Geometry check sheet. Reference: the model listing, model coordinates, mm. A direction names the side the tool comes from. Give positions to 0.01 mm unless a question says otherwise; leave off trailing zeros. Order: outer loops, then holes, each group sorted by start corner. A loop starts at its lowest first (then second) coordinate and runs counter-clockwise, first axis right, second up. Notation, with made-up numbers: M 26,-24.75 L 40,-24.75 A23 ccw 40,-15.75 Z; hole C 22,-21.5 d7. An arc over 180 degrees is marked long. One line per question, with ' | ' between items. Start each with the question number.
from build123d import *

# Parameters (mm, degrees)
SKETCH_1_W          = 50
SKETCH_1_H          = 50
EXTRUDE_1_DEPTH     = 3
SKETCH_2_W          = 50
SKETCH_2_H          = 50
SKETCH_2_W_2        = 44
SKETCH_2_H_2        = 44
EXTRUDE_2_DEPTH     = 17
SKETCH_3_W          = 4.5
SKETCH_3_H          = 2.5
CUT_EXTRUDE_1_DEPTH = 60.371710435
SKETCH_4_W          = 4.5
SKETCH_4_H          = 2.5
CUT_EXTRUDE_2_DEPTH = 60.371710435


with BuildPart() as part:
    # 草图1 → 凸台-拉伸1 (new body)
    with BuildSketch(Plane(origin=(0, 0, 0), x_dir=(1, 0, 0), z_dir=(0, 1, 0))):
        Rectangle(SKETCH_1_W, SKETCH_1_H)
    extrude(amount=EXTRUDE_1_DEPTH)

    # 草图2 → 凸台-拉伸2 (add)
    with BuildSketch(Plane(origin=(0, 3, 0), x_dir=(1, 0, 0), z_dir=(0, 1, 0))):
        Rectangle(SKETCH_2_W, SKETCH_2_H)
        Rectangle(SKETCH_2_W_2, SKETCH_2_H_2, mode=Mode.SUBTRACT)
    extrude(amount=EXTRUDE_2_DEPTH)

    # 草图3 → 切除-拉伸1 (cut, through all)
    with BuildSketch(Plane.XY.offset(25)):
        with Locations((-8, 17)):
            Rectangle(SKETCH_3_W, SKETCH_3_H)
        with Locations((8, 17)):
            Rectangle(SKETCH_3_W, SKETCH_3_H)
    extrude(amount=-CUT_EXTRUDE_1_DEPTH, mode=Mode.SUBTRACT)

    # 草图4 → 切除-拉伸2 (cut, through all)
    with BuildSketch(Plane(origin=(25, 0, 0), x_dir=(0, 0, -1), z_dir=(1, 0, 0))):
        with Locations((-8, 17)):
            Rectangle(SKETCH_4_W, SKETCH_4_H)
        with Locations((8, 17)):
            Rectangle(SKETCH_4_W, SKETCH_4_H)
    extrude(amount=-CUT_EXTRUDE_2_DEPTH, mode=Mode.SUBTRACT)


solid = part.part
Item 1: Cross-section at A-A, the plane x = -8. Record the cut outline in (y, z).
Item 2: Mould release check, pull along Y, two halves, no side actions. Record for faces 1 (the flat face through (-25, 10, 0)), 2 (the flat face through (0, 3, 0)), 3 (the flat face through (24, 17, 5.75)): released by +Y, released by -Y, zero draft, split by the parting line, or undercut.
Item 3: Set-up check for faces 4 (the flat face through (24, 15.75, 8)), 5 (the flat face through (-22.3, 20, -0.1)), 6 (the flat face through (-8, 18.25, 24)): record each of +Z, -Z, +X, -X, +Y, -Y from which the full face is reachable in a straight line by a thin tool's end or side.
Item 4: Cross-section at D-D, the plane y = 10.5. Record the cut outline in (x, z).
Item 5: Depth check by flat-ended pin: pin 1 (3.5 mm diameter, centred on x = 23, z = 7.5, fed in from -Y); pin 2 (13 mm diameter, centred on x = 0, z = 2.5, fed in from +Y). Enter the tip coordinate at first touch or a pass-through.
Item 6: Cross-section at C-C, the plane x = 15. Record the cut outline in (y, z), plus the area to 3 significant figures.
Item 7: Cross-section at B-B, the plane z = -7. Record the cut outline in (x, y), plus the area to 3 significant figures.
Item 8: Material ranges on line 1 along X through (y, z) = (9.5, 12); line 2 along Y through (x, z) = (-1.5, -19), recorded low to high.
Outcome:
1) outline: M 0,-25 L 15.75,-25 L 15.75,-22 L 3,-22 L 3,22 L 15.75,22 L 15.75,25 L 0,25 Z; M 18.25,-25 L 20,-25 L 20,-22 L 18.25,-22 Z; M 18.25,22 L 20,22 L 20,25 L 18.25,25 Z
2) face 1: zero draft | face 2: released by +Y | face 3: undercut
3) face 4: +X, -X | face 5: +Z, -Z, +X, -X, +Y | face 6: +Z, -Z
4) outline: M -25,-25 L 25,-25 L 25,25 L -25,25 Z; hole M -22,-22 L 22,-22 L 22,22 L -22,22 Z
5) pin 1: stops at y = 0 | pin 2: stops at y = 3
6) outline: M 0,-25 L 20,-25 L 20,-22 L 3,-22 L 3,22 L 20,22 L 20,25 L 0,25 Z | area: 252 mm²
7) outline: M -25,0 L 25,0 L 25,15.75 L 22,15.75 L 22,3 L -22,3 L -22,15.75 L -25,15.75 Z; M -25,18.25 L -22,18.25 L -22,20 L -25,20 Z; M 22,18.25 L 25,18.25 L 25,20 L 22,20 Z | area: 237 mm²
8) line 1: x = -25 to -22, 22 to 25 | line 2: y = 0 to 3
